```python
from build123d import *

# Parameters (mm, degrees)
F0_R     = 11.5
F1_DEPTH = 2
F2_R     = 5.25
F3_DEPTH = 0.7
F4_R     = 4
F5_DEPTH = 3
F6_R     = 1.5


with BuildPart() as f1:
    # F0 (on Top) → F1 (new body)
    with BuildSketch(Plane.XY):
        Circle(F0_R)
    extrude(amount=F1_DEPTH)

    # F2 (on face) → F3 (join)
    with BuildSketch(Plane.XY.offset(2)):
        Circle(F2_R)
    extrude(amount=F3_DEPTH)

    # F4 (on face) → F5 (join)
    with BuildSketch(Plane.XY.offset(2.7)):
        Circle(F4_R)
    extrude(amount=F5_DEPTH)

    # F6
    f6_edges = [f1.edges().sort_by_distance(p)[0] for p in [
        (-11.5, 0, 0),
    ]]
    fillet(f6_edges, radius=F6_R)


solid = f1.part
```
CAD build for the part. Positions are in the model's coordinates, mm. A direction names the side the tool comes from. Round coordinates to 2 decimals unless told otherwise and drop trailing zeros. Loops run counter-clockwise (first coordinate to the right, second up) from the corner with the lowest first, then second, coordinate; pieces in that order, holes last. Notation, with made-up numbers: (30, -20) - (86, -20) arc R22 cw to (86, 12) - close; hole circle Ø7 at (82.5, 32). An arc over 180 degrees is marked (long way). Return JSON: item names as keys, results as strings. Group by question number.
Q1. Band-saw the part on A-A on x = 0. Give the cut face in (y, z).
Q2. Flat gauge pins, fed straight in: pin 1 Ø3 at (x, z) = (1.5, 0.5) entering from +Y; pin 2 Ø1 at (y, z) = (1, 0.5) entering from -X; pin 3 Ø6 at (x, y) = (9, 6) entering from +Z. Where does each tip first touch, or does it go through?
Q3. Drill centre lines: line 1 along Z through (x, y) = (3.25, 3); line 2 along Z through (x, y) = (-4.5, -6.75); line 3 along Y through (x, z) = (3.5, 0.95). Where is each one in solid material? Low to high. Write a range as [from, to].
Q4. Tool access for faces 1 (the face through (0, 0, 0)), 2 (the face through (-0.867, -3.905, 4.179)): list every direction of +Z, -Z, +X, -X, +Y, -Y with a clear straight run to the whole face (end or side of a thin tool).
Solutions:
{
 "1": {"outline": "(-11.5, 1.5) arc R1.5 ccw to (-10, 0) - (10, 0) arc R1.5 ccw to (11.5, 1.5) - (11.5, 2) - (5.25, 2) - (5.25, 2.7) - (4, 2.7) - (4, 5.7) - (-4, 5.7) - (-4, 2.7) - (-5.25, 2.7) - (-5.25, 2) - (-11.5, 2) - close"},
 "2": {"pin 1": "stops at y = 11.49", "pin 2": "stops at x = -11.38", "pin 3": "stops at z = 2"},
 "3": {"line 1": "z = [0, 2.7]", "line 2": "z = [0, 2]", "line 3": "y = [-10.84, 10.84]"},
 "4": {"face 1": "-Z, +X, -X, +Y, -Y", "face 2": "+Z"}
}
